Build history of the part. All positions in model axes, mm. Face numbers are marked on the shaded views. A direction names the side the tool comes from. Round coordinates to 2 decimals unless told otherwise and drop trailing zeros. Write each loop counter-clockwise with the first axis right and the second up, starting at its lowest first coordinate (ties: lowest second). Pieces come first, ordered by that corner, then holes.
Item 1: 3-axis set-ups, long thin cutter, end or side, ignore diameter. For the marked faces 1, 2 and 3: which of +Z, -Z, +X, -X, +Y, -Y reach the whole face in a straight line?
Item 2: Band-saw the part on B-B, the plane x = -5.25. Write the cut outline in (y, z), then the cut area to 3 significant figures.
Item 3: Band-saw the part on D-D, the plane z = -5. Write the cut outline in (x, y), then the cut area to 3 significant figures.
Item 4: Drop flat-ended pins along their axis: pin 1 Ø1.4 at (y, z) = (-0.5, -5) entering from +X; pin 2 Ø1.5 at (y, z) = (0.5, -5.5) entering from -X; pin 3 Ø1 at (x, y) = (-2, -0.5) entering from -Z. Give the stop position or say it passes through.
Item 5: Wall check: probe 1 along Y at (x, z) = (9.8, 4.75); probe 2 along X at (y, z) = (-1.4, -4.5); probe 3 along X at (y, z) = (-0.85, 6). Give the ranges that are in metal, low to high.
Item 6: Band-saw the part on A-A, the plane z = -2.75. Write the cut outline in (x, y), then the cut area to 3 significant figures.
Item 7: Band-saw the part on C-C, the plane z = 4.75. Write the cut outline in (x, y), then the cut area to 3 significant figures.
Item 8: Mould opens along X. For the marked faces 4, 5 and 6 say: +X half, -X half, draft (parallel to the pull), parting line (faces both ways), or undercut.
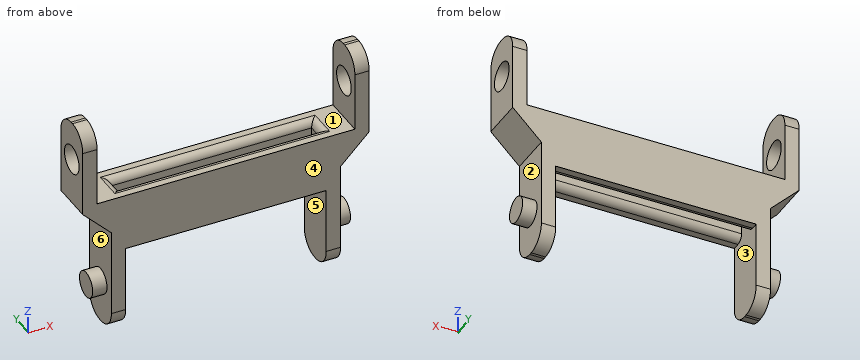
```python
from build123d import *

# Parameters (mm, degrees)
SKETCH1_W           = 16
SKETCH1_H           = 3
SKETCH1_W_2         = 14
SKETCH1_H_2         = 1
EXTRUDE_THIN1_DEPTH = 2
SKETCH2_W           = 6
SKETCH2_H           = 3
BOSS_EXTRUDE1_DEPTH = 2
CHAMFER3_SIZE       = 2
SKETCH3_W           = 5.5
SKETCH3_H           = 3
CUT_EXTRUDE1_DEPTH  = 1
BOSS_EXTRUDE2_START = -1
SKETCH4_W           = 6
SKETCH4_H           = 3
BOSS_EXTRUDE2_DEPTH = 1
SKETCH5_W           = 6
SKETCH5_H           = 3
BOSS_EXTRUDE3_DEPTH = 1
CHAMFER4_SIZE       = 2
FILLET1_R           = 1.4
SKETCH7_R           = 1
CUT_EXTRUDE3_DEPTH  = 1
SKETCH8_R           = 0.9
BOSS_EXTRUDE5_DEPTH = 2
FILLET4_R           = 0.5
FILLET6_R           = 0.5


with BuildPart() as part:
    # Sketch1 → Extrude-Thin1 (new, symmetric)
    with BuildSketch(Plane.XY):
        Rectangle(SKETCH1_W, SKETCH1_H)
        Rectangle(SKETCH1_W_2, SKETCH1_H_2, mode=Mode.SUBTRACT)
    extrude(amount=EXTRUDE_THIN1_DEPTH, both=True)

    # Sketch2 → Boss-Extrude1 (add)
    with BuildSketch(Plane(origin=(8, 0, 0), x_dir=(0, 0, -1), z_dir=(1, 0, 0))):
        with Locations((-4.5, 0)):
            Rectangle(SKETCH2_W, SKETCH2_H)
    boss_extrude1 = extrude(amount=BOSS_EXTRUDE1_DEPTH)

    # Chamfer3
    chamfer3_edges = [part.edges().sort_by_distance(p)[0] for p in [
        (8, 0, 1.5),
    ]]
    chamfer(chamfer3_edges, length=CHAMFER3_SIZE - 0.0001)  # a hair under: the kernel refuses the full size

    # Sketch3 → Cut-Extrude1 (cut)
    with BuildSketch(Plane.ZY.offset(-8)):
        with Locations((4.75, 0)):
            Rectangle(SKETCH3_W, SKETCH3_H)
    cut_extrude1 = extrude(amount=-CUT_EXTRUDE1_DEPTH, mode=Mode.SUBTRACT)

    # Sketch4 → Boss-Extrude2 (add)
    with BuildSketch(Plane(origin=(8, 0, 0), x_dir=(0, 0, -1), z_dir=(1, 0, 0)).offset(BOSS_EXTRUDE2_START)):
        with Locations((5, 0)):
            Rectangle(SKETCH4_W, SKETCH4_H)
    extrude(amount=BOSS_EXTRUDE2_DEPTH)

    # Mirror2: Boss-Extrude1, Cut-Extrude1 across plane
    add(boss_extrude1.mirror(Plane(origin=(0, 0, 0), x_dir=(0, 0, 1), z_dir=(1, 0, 0))))
    add(cut_extrude1.mirror(Plane(origin=(0, 0, 0), x_dir=(0, 0, 1), z_dir=(1, 0, 0))), mode=Mode.SUBTRACT)

    # Sketch5 → Boss-Extrude3 (add)
    with BuildSketch(Plane.ZY.offset(8)):
        with Locations((-5, 0)):
            Rectangle(SKETCH5_W, SKETCH5_H)
    extrude(amount=-BOSS_EXTRUDE3_DEPTH)

    # Chamfer4
    chamfer4_edges = [part.edges().sort_by_distance(p)[0] for p in [
        (-8, 0, 1.5),
    ]]
    chamfer(chamfer4_edges, length=CHAMFER4_SIZE - 0.0001)  # a hair under: the kernel refuses the full size

    # Fillet1
    fillet1_edges = [part.edges().sort_by_distance(p)[0] for p in [
        (-7.5, 1.5, -8),
        (-7.5, -1.5, -8),
        (9.5, 1.5, 7.5),
        (9.5, -1.5, 7.5),
        (7.5, -1.5, -8),
        (7.5, 1.5, -8),
        (-9.5, -1.5, 7.5),
        (-9.5, 1.5, 7.5),
    ]]
    fillet(fillet1_edges, radius=FILLET1_R)

    # Sketch7 → Cut-Extrude3 (cut)
    with BuildSketch(Plane.ZY.offset(-9)):
        with Locations((4.75, 0)):
            Circle(SKETCH7_R)
    cut_extrude3 = extrude(amount=-CUT_EXTRUDE3_DEPTH, mode=Mode.SUBTRACT)

    # Mirror6: Cut-Extrude3 across plane
    add(cut_extrude3.mirror(Plane(origin=(0, 0, 0), x_dir=(0, 0, 1), z_dir=(1, 0, 0))), mode=Mode.SUBTRACT)

    # Sketch8 → Boss-Extrude5 (add)
    with BuildSketch(Plane(origin=(-7, 0, 0), x_dir=(0, 0, -1), z_dir=(1, 0, 0))):
        with Locations((5, 0)):
            Circle(SKETCH8_R)
    boss_extrude5 = extrude(amount=-BOSS_EXTRUDE5_DEPTH)

    # Mirror7: Boss-Extrude5 across plane
    add(boss_extrude5.mirror(Plane(origin=(0, 0, 0), x_dir=(0, 0, 1), z_dir=(1, 0, 0))))

    # Fillet4
    fillet4_edges = [part.edges().sort_by_distance(p)[0] for p in [
        (0, -0.5, -2),
        (0, 0.5, -2),
    ]]
    fillet(fillet4_edges, radius=FILLET4_R)

    # Fillet6
    fillet6_edges = [part.edges().sort_by_distance(p)[0] for p in [
        (-7, 0, 2),
        (0, -0.5, 2),
        (7, 0, 2),
        (0, 0.5, 2),
    ]]
    fillet(fillet6_edges, radius=FILLET6_R)


solid = part.part
```
Results:
1. face 1: +Z, +Y, -Y
1. face 2: +X
1. face 3: -Z
2. outline: (-1.5, -2) - (-1, -2) arc R0.5 ccw to (-0.5, -1.5) - (-0.5, 1.5) arc R0.5 ccw to (-1, 2) - (-1.5, 2) - close; (0.5, -1.5) arc R0.5 ccw to (1, -2) - (1.5, -2) - (1.5, 2) - (1, 2) arc R0.5 ccw to (0.5, 1.5) - close
2. area: 7.79 mm2
3. outline: (-9, -0.9) - (-8, -0.9) - (-8, -1.5) - (-7, -1.5) - (-7, 1.5) - (-8, 1.5) - (-8, 0.9) - (-9, 0.9) - close; (7, -1.5) - (8, -1.5) - (8, -0.9) - (9, -0.9) - (9, 0.9) - (8, 0.9) - (8, 1.5) - (7, 1.5) - close
3. area: 9.60 mm2
4. pin 1: stops at x = 9
4. pin 2: stops at x = -9
4. pin 3: stops at z = -2
5. probe 1: y = -1.5 to -1, 1 to 1.5
5. probe 2: x = -8 to -7, 7 to 8
5. probe 3: x = -10 to -9, 9 to 10
6. outline: (-8, -1.5) - (-7, -1.5) - (-7, 1.5) - (-8, 1.5) - close; (7, -1.5) - (8, -1.5) - (8, 1.5) - (7, 1.5) - close
6. area: 6.00 mm2
7. outline: (-10, -1.5) - (-9, -1.5) - (-9, -1) - (-10, -1) - close; (-10, 1) - (-9, 1) - (-9, 1.5) - (-10, 1.5) - close; (9, -1.5) - (10, -1.5) - (10, -1) - (9, -1) - close; (9, 1) - (10, 1) - (10, 1.5) - (9, 1.5) - close
7. area: 2.00 mm2
8. face 4: draft
8. face 5: undercut
8. face 6: -X half
